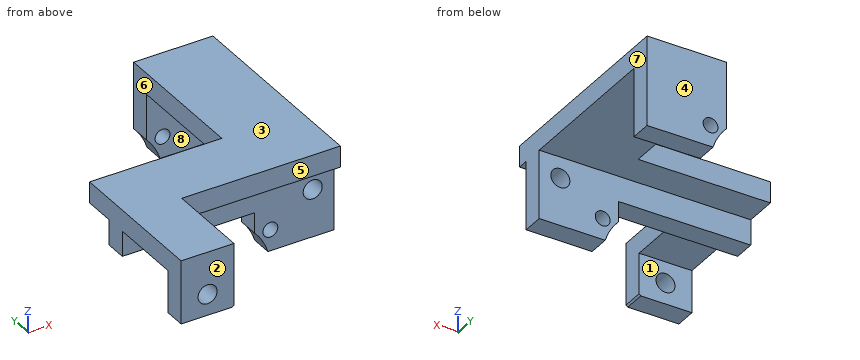
```python
from build123d import *

# Parameters (mm, degrees)
PAD_DEPTH       = 4
SKETCH001_W     = 25
SKETCH001_H     = 4
PAD001_DEPTH    = 4.8
SKETCH002_W     = 15
SKETCH002_H     = 4
PAD002_DEPTH    = 13
SKETCH003_W     = 10
SKETCH003_H     = 4
PAD003_DEPTH    = 8
SKETCH004_R     = 1.4
SKETCH004_R_2   = 11
POCKET_DEPTH    = 100
SKETCH005_R     = 1.8
POCKET001_DEPTH = 5
SKETCH007_R     = 1.8
POCKET002_DEPTH = 5
SKETCH008_W     = 25
SKETCH008_H     = 4
PAD004_DEPTH    = 6


with BuildPart() as part:
    # Sketch → Pad (new body)
    with BuildSketch(Plane.XY):
        Polygon((0, 33), (0, 0), (-25, 0), (-25, -22), (-15, -22), (-15, -6), (15, -6), (15, 33), align=None)
    extrude(amount=PAD_DEPTH)

    # Sketch001 (on Face9 of Pad) → Pad001 (join)
    with BuildSketch(Plane(origin=(0, 0, 0), x_dir=(1, 0, 0), z_dir=(0, 0, -1))):
        with Locations((-12.5, 2)):
            Rectangle(SKETCH001_W, SKETCH001_H)
    extrude(amount=PAD001_DEPTH)

    # Sketch002 (on Face4 of Pad001) → Pad002 (join)
    with BuildSketch(Plane(origin=(0, 0, 0), x_dir=(1, 0, 0), z_dir=(0, 0, -1))):
        with Locations((7.5, -31)):
            Rectangle(SKETCH002_W, SKETCH002_H)
        with Locations((7.5, 2)):
            Rectangle(SKETCH002_W, SKETCH002_H)
    extrude(amount=PAD002_DEPTH)

    # Sketch003 (on Face4 of Pad002) → Pad003 (join)
    with BuildSketch(Plane(origin=(0, 0, 0), x_dir=(1, 0, 0), z_dir=(0, 0, -1))):
        with Locations((-20, 20)):
            Rectangle(SKETCH003_W, SKETCH003_H)
    extrude(amount=PAD003_DEPTH)

    # Sketch004 (on Face20 of Pad003) → Pocket (cut)
    with BuildSketch(Plane(origin=(0, 33, 0), x_dir=(-1, 0, 0), z_dir=(0, 1, 0))):
        with Locations((-3, -9)):
            Circle(SKETCH004_R)
        with Locations((8, -16.2)):
            Circle(SKETCH004_R_2)
    extrude(amount=-POCKET_DEPTH, mode=Mode.SUBTRACT)

    # Sketch005 (on Face18 of Pocket) → Pocket001 (cut)
    with BuildSketch(Plane.XZ.offset(22)):
        with Locations((-20, -4)):
            Circle(SKETCH005_R)
    extrude(amount=-POCKET001_DEPTH, mode=Mode.SUBTRACT)

    # Sketch007 (on Face15 of Pocket001) → Pocket002 (cut)
    with BuildSketch(Plane.XZ.offset(4)):
        with Locations((11, -4)):
            Circle(SKETCH007_R)
    extrude(amount=-POCKET002_DEPTH, mode=Mode.SUBTRACT)

    # Sketch008 (on Face17 of Pocket002) → Pad004 (join)
    with BuildSketch(Plane(origin=(0, 0, 0), x_dir=(-1, 0, 0), z_dir=(0, 1, 0))):
        with Locations((12.5, 2)):
            Rectangle(SKETCH008_W, SKETCH008_H)
    extrude(amount=PAD004_DEPTH)


solid = part.part
```
For this review, take the finished solid that the model builds, in its own axes (mm). Face numbers are marked on the shaded views. A direction names the side the tool comes from. Coordinates: 2 decimals unless noted, no trailing zeros. Write each loop counter-clockwise with the first axis right and the second up, starting at its lowest first coordinate (ties: lowest second). Pieces come first, ordered by that corner, then holes.
(1) Add section C-C on z = -4. Give the boundary of the cut face in (x, y), then the cut area to 3 significant figures.
(2) Add section D-D on x = -8. Give the boundary of the cut face in (y, z), then the cut area to 3 significant figures.
(3) The part is to be moulded in two halves that separate along Y. For the marked faces 1, 2 and 3, say which applies: +Y half, -Y half, draft (parallel to the pull), parting line (faces both ways), or undercut.
(4) Tool access review of the marked faces 4, 5, 6, 7 and 8: name each direction out of +Z, -Z, +X, -X, +Y, -Y from which nothing blocks a thin tool from reaching the whole face with its end or side.
(5) Add section B-B on x = -20. Give the boundary of the cut face in (y, z), then the cut area to 3 significant figures.
(6) Add section A-A on z = -6.5. Give the boundary of the cut face in (x, y), then the cut area to 3 significant figures.
(7) Wall thickness on probe 1 along Y at (x, z) = (7, -5.5); probe 2 along Z at (x, y) = (3, 31); probe 3 along X at (y, z) = (-17, 3.5): over which ranges is each line inside the solid? List them lowest first.
(8) For pin 1 Ø14.5 at (x, y) = (-8.5, 15.5) entering from -Z; pin 2 Ø4 at (x, z) = (-18.5, -5.5) entering from +Y; pin 3 Ø3 at (y, z) = (-1.5, -7.5) entering from -X; pin 4 Ø4 at (x, z) = (8.5, -4.5) entering from -Y, all flat-tipped, find the tip position at first contact; note any pin that passes through.
Answer sheet:
1. outline: (-25, -22) - (-21.8, -22) - (-21.8, -18) - (-25, -18) - close; (-25, -4) - (9.2, -4) - (9.2, 0) - (-25, 0) - close; (-18.2, -22) - (-15, -22) - (-15, -18) - (-18.2, -18) - close; (0, 29) - (15, 29) - (15, 33) - (0, 33) - close; (12.8, -4) - (15, -4) - (15, 0) - (12.8, 0) - close
1. area: 231 mm2
2. outline: (-6, 0) - (-4, 0) - (-4, -4.8) - (0, -4.8) - (0, 0) - (6, 0) - (6, 4) - (-6, 4) - close
2. area: 67.2 mm2
3. face 1: undercut
3. face 2: -Y half
3. face 3: draft
4. face 4: +Z, -Z, +X, -X, +Y
4. face 5: +Z, -Z, +X, -Y
4. face 6: +Z, -Z, -X, +Y
4. face 7: +Z, -Z, +X, +Y, -Y
4. face 8: -Z, +X, -X
5. outline: (-22, -8) - (-18, -8) - (-18, -5.8) - (-22, -5.8) - close; (-22, -2.2) - (-18, -2.2) - (-18, 0) - (-4, 0) - (-4, -4.8) - (0, -4.8) - (0, 0) - (6, 0) - (6, 4) - (-22, 4) - close
5. area: 149 mm2
6. outline: (-25, -22) - (-15, -22) - (-15, -18) - (-25, -18) - close; (0, -4) - (15, -4) - (15, 0) - (0, 0) - close; (0, 29) - (15, 29) - (15, 33) - (0, 33) - close
6. area: 160 mm2
7. probe 1: y = -4 to 0, 29 to 33
7. probe 2: z = -13 to -10.4, -7.6 to 4
7. probe 3: x = -25 to -15
8. pin 1: passes through
8. pin 2: stops at y = 0
8. pin 3: stops at x = 0
8. pin 4: stops at y = -4
